from build123d import *

# Parameters (mm, degrees)
SKETCH1_R           = 4
BOSS_EXTRUDE2_DEPTH = 4.8
SKETCH2_R           = 30
SKETCH2_R_2         = 4
BOSS_EXTRUDE3_DEPTH = 12
SKETCH3_R           = 1.75
CUT_EXTRUDE1_DEPTH  = 16.8
SKETCH4_R           = 3
CUT_EXTRUDE2_DEPTH  = 2


with BuildPart() as part:
    # Sketch1 → Boss-Extrude2 (new body)
    with BuildSketch(Plane(origin=(0, 0, 0), x_dir=(1, 0, 0), z_dir=(0, 1, 0))):
        Polygon((86.602540378, 0), (43.301270189, 75), (-43.301270189, 75), (-86.602540378, 0), (-43.301270189, -75), (43.301270189, -75), align=None)
        with Locations(Location((0, 0, 0), (0, 0, 270))):
            Circle(SKETCH1_R, mode=Mode.SUBTRACT)
    extrude(amount=BOSS_EXTRUDE2_DEPTH)

    # Sketch2 → Boss-Extrude3 (add)
    with BuildSketch(Plane(origin=(0, 4.8, 0), x_dir=(1, 0, 0), z_dir=(0, 1, 0))):
        with Locations(Location((0, 0, 0), (0, 0, 270))):
            Circle(SKETCH2_R)
        with Locations(Location((0, 0, 0), (0, 0, 270))):
            Circle(SKETCH2_R_2, mode=Mode.SUBTRACT)
    extrude(amount=BOSS_EXTRUDE3_DEPTH)

    # Sketch3 → Cut-Extrude1 (cut)
    with BuildSketch(Plane(origin=(0, 16.8, 0), x_dir=(1, 0, 0), z_dir=(0, 1, 0))):
        with Locations(Location((25, 0, 0), (0, 0, 270))):
            Circle(SKETCH3_R)
        with Locations(Location((0, -25, 0), (0, 0, 270))):
            Circle(SKETCH3_R)
        with Locations(Location((-25, 0, 0), (0, 0, 270))):
            Circle(SKETCH3_R)
        with Locations(Location((0, 25, 0), (0, 0, 270))):
            Circle(SKETCH3_R)
        with Locations(Location((40, 69.282032303, 0), (0, 0, 270))):
            Circle(SKETCH3_R)
        with Locations(Location((80, 0, 0), (0, 0, 270))):
            Circle(SKETCH3_R)
        with Locations(Location((40, -69.282032303, 0), (0, 0, 270))):
            Circle(SKETCH3_R)
        with Locations(Location((-40, -69.282032303, 0), (0, 0, 270))):
            Circle(SKETCH3_R)
        with Locations(Location((-80, 0, 0), (0, 0, 270))):
            Circle(SKETCH3_R)
        with Locations(Location((-40, 69.282032303, 0), (0, 0, 270))):
            Circle(SKETCH3_R)
    extrude(amount=-CUT_EXTRUDE1_DEPTH, mode=Mode.SUBTRACT)

    # Sketch4 → Cut-Extrude2 (cut)
    with BuildSketch(Plane(origin=(0, 16.8, 0), x_dir=(1, 0, 0), z_dir=(0, 1, 0))):
        with Locations(Location((0, 25, 0), (0, 0, 270))):
            Circle(SKETCH4_R)
        with Locations(Location((25, 0, 0), (0, 0, 270))):
            Circle(SKETCH4_R)
        with Locations(Location((0, -25, 0), (0, 0, 270))):
            Circle(SKETCH4_R)
        with Locations(Location((-25, 0, 0), (0, 0, 270))):
            Circle(SKETCH4_R)
    extrude(amount=-CUT_EXTRUDE2_DEPTH, mode=Mode.SUBTRACT)


solid = part.part
Design review of the part built by this model. Coordinates are the model's own, in mm. A direction names the side the tool comes from. Coordinates: 2 decimals unless noted, no trailing zeros. Loops run counter-clockwise (first coordinate to the right, second up) from the corner with the lowest first, then second, coordinate; pieces in that order, holes last.
Item 1: Add section C-C (z = -16.5). Write out the cut boundary in (x, y), and give its area (3 significant figures).
Completed:
outline: (-77.08, 0) - (77.08, 0) - (77.08, 4.8) - (25.05, 4.8) - (25.05, 16.8) - (-25.05, 16.8) - (-25.05, 4.8) - (-77.08, 4.8) - close
area: 1,340 mm2
Item 2: Add section D-D (x = -34). Write out the cut boundary in (y, z), and give its area (3 significant figures).
Completed:
outline: (0, -75) - (4.8, -75) - (4.8, 75) - (0, 75) - close
area: 720 mm2
Item 3: Draft analysis for pull direction X (two halves, no side actions). For faces 3 (the cylindrical face through (-81.71, 2.43, -0.38)), 4 (the cylindrical face through (1.32, 10.72, -29.97)), 5 (the flat face through (65.255, 2.366, -36.975)), state which applies: pulls with the +X half, pulls with the -X half, needs draft (parallel to the pull), parting line crosses it, or undercut.
Completed:
face 3: undercut
face 4: parting line crosses it
face 5: pulls with the +X half
Item 4: Clearance check with flat-ended pins moving along their axes: pin 1 (6 mm diameter, centred on x = -12.5, y = 10, fed in from -Z); pin 2 (1.8 mm diameter, centred on x = 1, z = 24, fed in from +Y); pin 3 (6 mm diameter, centred on x = -10.5, y = 12.5, fed in from +Z). State where each tip first meets the part, or that it passes through.
Completed:
pin 1: stops at z = -28.46
pin 2: stops at y = 14.8
pin 3: stops at z = 29.05
Item 5: Add section A-A (y = 2). Give the number of separate pieces and of enclosed holes in the cut face, and give its area (3 significant figures).
Completed:
separate pieces: 1
enclosed holes: 11
area: 19,300 mm2
Item 6: Wall thickness on L1, parallel to X at y = 1.45, z = 0; L2, parallel to X at y = 5.25, z = 0; L3, parallel to X at y = 7.5, z = 2.5: over which ranges is each line inside the solid? List them lowest first.
Completed:
L1: x = -86.6 to -81.75, -78.25 to -26.75, -23.25 to -4, 4 to 23.25, 26.75 to 78.25, 81.75 to 86.6
L2: x = -30 to -26.75, -23.25 to -4, 4 to 23.25, 26.75 to 30
L3: x = -29.9 to -3.12, 3.12 to 29.9
Item 7: Add section B-B (x = -9). Write out the cut boundary in (y, z), and give its area (3 significant figures).
Completed:
outline: (0, -75) - (4.8, -75) - (4.8, -28.62) - (16.8, -28.62) - (16.8, 28.62) - (4.8, 28.62) - (4.8, 75) - (0, 75) - close
area: 1,410 mm2
Item 8: For faces 1 (the cylindrical face through (39.33, 2.43, 70.9)), 2 (the flat face through (25, 14.8, 2)), list the 3-axis set-ups (+Z, -Z, +X, -X, +Y, -Y) from which the entire face can be reached by the end or side of a thin tool; tool diameter is ignored.
Completed:
face 1: +Y, -Y
face 2: +Y
